```python
from build123d import *

# Parameters (mm, degrees)
SKETCH1_W                     = 50.8
SKETCH1_H                     = 50.8
BOSS_EXTRUDE1_DEPTH           = 50.8
F_1_4_CLEARANCE_HOLE1_D       = 6.7564
SKETCH4_R                     = 2.54
CUT_EXTRUDE1_DEPTH            = 63.217039467
TAP_DRILL_FOR_8_32_TAP1_D     = 3.4544
TAP_DRILL_FOR_8_32_TAP1_DEPTH = 12.7
TAP_DRILL_FOR_8_32_TAP1_TIP   = 1.037806461


with BuildPart() as part:
    # Sketch1 → Boss-Extrude1 (new body)
    with BuildSketch(Plane(origin=(0, 0, 0), x_dir=(1, 0, 0), z_dir=(0, 1, 0))):
        Rectangle(SKETCH1_W, SKETCH1_H)
    extrude(amount=BOSS_EXTRUDE1_DEPTH)

    # 1/4 Clearance Hole1 (through all)
    with Locations(Plane(origin=(0, 50.8, 0), x_dir=(1, 0, 0), z_dir=(0, 1, 0))):
        with Locations((-19.05, 19.05), (19.05, 19.05), (0, -19.05)):
            Hole(F_1_4_CLEARANCE_HOLE1_D / 2)

    # Sketch4 → Cut-Extrude1 (cut, through all)
    with BuildSketch(Plane(origin=(0, 50.8, 0), x_dir=(1, 0, 0), z_dir=(0, 1, 0))):
        with Locations(Location((0, 0, 0), (0, 0, 270))):
            Circle(SKETCH4_R)
    extrude(amount=-CUT_EXTRUDE1_DEPTH, mode=Mode.SUBTRACT)

    # Tap Drill for #8-32 Tap1
    with Locations(Plane(origin=(0, 50.8, 0), x_dir=(1, 0, 0), z_dir=(0, 1, 0))):
        with Locations((-12.7, 0), (12.7, 0)):
            Hole(TAP_DRILL_FOR_8_32_TAP1_D / 2, depth=TAP_DRILL_FOR_8_32_TAP1_DEPTH)
            with Locations((0, 0, -(TAP_DRILL_FOR_8_32_TAP1_DEPTH + TAP_DRILL_FOR_8_32_TAP1_TIP / 2))):  # 118° drill point
                Cone(0, TAP_DRILL_FOR_8_32_TAP1_D / 2, TAP_DRILL_FOR_8_32_TAP1_TIP, mode=Mode.SUBTRACT)


solid = part.part
```
Design review of the part built by this model. Coordinates are the model's own, in mm. A direction names the side the tool comes from. Coordinates: 2 decimals unless noted, no trailing zeros. Write each loop counter-clockwise with the first axis right and the second up, starting at its lowest first coordinate (ties: lowest second). Pieces come first, ordered by that corner, then holes.
1) Insertion check: pin 1 (1 mm diameter, centred on x = 2.5, z = 2, fed in from -Y). The pin has a flat end and moves straight along its axis. Give the tip position at first contact, or say it passes through.
2) Add section D-D (z = -19.05). Write out the cut boundary in (x, y).
3) Add section C-C (x = -19.05). Write out the cut boundary in (y, z).
4) Add section B-B (z = 19.05). Write out the cut boundary in (x, y).
5) Mouldability with a two-part tool opening along X and no side actions: class faces 1 (the flat face through (0, 25, 25.4)), 2 (the flat face through (-25.4, 25, 0)), 3 (the cylindrical face through (0.44, 25.04, 15.7)), 4 (the flat face through (25.4, 25, 0)) as +X half, -X half, draft (parallel to the pull), parting line (faces both ways), or undercut.
6) To check wall thickness, follow L1, parallel to X at y = 37, z = 0; L2, parallel to Z at x = -1.5, y = 14; L3, parallel to X at y = 13.5, z = 19.05. State the ranges of each line that lie inside material, in increasing order.
7) Add section A-A (y = 6). Write out the cut boundary in (x, z).
8) Machinability: for faces 5 (the cylindrical face through (11.105, 44.361, 0.662)), 6 (the flat face through (0, 0, -6)), which of the approach directions +Z, -Z, +X, -X, +Y, -Y give a long, thin tool a straight path to every point of the face, cutting with its end or side? Answer none if there is none.
Check result:
1. pin 1: stops at y = 0
2. outline: (-25.4, 0) - (-22.43, 0) - (-22.43, 50.8) - (-25.4, 50.8) - close; (-15.67, 0) - (15.67, 0) - (15.67, 50.8) - (-15.67, 50.8) - close; (22.43, 0) - (25.4, 0) - (25.4, 50.8) - (22.43, 50.8) - close
3. outline: (0, -25.4) - (50.8, -25.4) - (50.8, -22.43) - (0, -22.43) - close; (0, -15.67) - (50.8, -15.67) - (50.8, 25.4) - (0, 25.4) - close
4. outline: (-25.4, 0) - (-3.38, 0) - (-3.38, 50.8) - (-25.4, 50.8) - close; (3.38, 0) - (25.4, 0) - (25.4, 50.8) - (3.38, 50.8) - close
5. face 1: draft
5. face 2: -X half
5. face 3: undercut
5. face 4: +X half
6. L1: x = -25.4 to -2.54, 2.54 to 25.4
6. L2: z = -25.4 to -2.05, 2.05 to 16.02, 22.08 to 25.4
6. L3: x = -25.4 to -3.38, 3.38 to 25.4
7. outline: (-25.4, -25.4) - (25.4, -25.4) - (25.4, 25.4) - (-25.4, 25.4) - close; hole circle Ø6.76 at (-19.05, -19.05); hole circle Ø6.76 at (0, 19.05); hole circle Ø5.08 at (0, 0); hole circle Ø6.76 at (19.05, -19.05)
8. face 5: +Y
8. face 6: +Z, -Z, +X, -X, -Y
